Source: CAD feature listing. Evaluate the final solid. Frame: model axes, mm. A direction names the side the tool comes from. Give positions to 0.01 mm unless a question says otherwise; leave off trailing zeros. Loops run counter-clockwise (first coordinate to the right, second up) from the corner with the lowest first, then second, coordinate; pieces in that order, holes last. Notation, with made-up numbers: M 82.25,65.5 L 94.25,65.5 A25 ccw 94.25,98.5 Z; hole C -2,63 d1. An arc over 180 degrees is marked long. Put each result on its own line as item: value.
from build123d import *

# Parameters (mm, degrees)
BOSS_EXTRUDE1_DEPTH = 5
SKETCH5_R           = 2
CUT_EXTRUDE1_DEPTH  = 1.5
SKETCH2_W           = 3
SKETCH2_H           = 3
CUT_EXTRUDE2_DEPTH  = 10


with BuildPart() as part:
    # Sketch1 → Boss-Extrude1 (new body)
    with BuildSketch(Plane.XY):
        with BuildLine():
            ThreePointArc((-10.997222353, 0.247207602), (-0.699194891, -10.977755935), (10.939721705, -1.149999502))
            ThreePointArc((10.939721705, -1.149999502), (10.984920466, -0.575788859), (11.000000502, 4.98e-07))
            ThreePointArc((11.000000502, 4.98e-07), (10.991774906, 0.425318543), (10.967110422, 0.850000498))
            ThreePointArc((10.967110422, 0.850000498), (-0.301772264, 10.995860878), (-10.997222353, 0.247207602))
        make_face()
        with BuildLine():
            ThreePointArc((4.98e-07, -9.049999502), (1.050000497, -7.999999502), (4.96e-07, -6.949999502))
            ThreePointArc((4.96e-07, -6.949999502), (-1.049999502, -7.999999503), (4.98e-07, -9.049999502))
        make_face(mode=Mode.SUBTRACT)
        with BuildLine():
            ThreePointArc((8.000000496, 1.050000498), (6.950000497, 4.97e-07), (8.000000498, -1.049999502))
            ThreePointArc((8.000000498, -1.049999502), (9.050000498, 4.98e-07), (8.000000496, 1.050000498))
        make_face(mode=Mode.SUBTRACT)
        with BuildLine():
            ThreePointArc((4.96e-07, 9.050000498), (-1.049999503, 8.000000497), (4.98e-07, 6.950000498))
            ThreePointArc((4.98e-07, 6.950000498), (1.050000498, 8.000000498), (4.96e-07, 9.050000498))
        make_face(mode=Mode.SUBTRACT)
        with BuildLine():
            ThreePointArc((-9.049999498, -9.4808e-05), (-8.742427926, -0.742495317), (-7.999999502, -1.049999502))
            ThreePointArc((-7.999999502, -1.049999502), (-6.949999502, 4.95e-07), (-7.999999497, 1.050000498))
            ThreePointArc((-7.999999497, 1.050000498), (-8.742495315, 0.742428924), (-9.049999498, -9.4808e-05))
        make_face(mode=Mode.SUBTRACT)
    extrude(amount=BOSS_EXTRUDE1_DEPTH)

    # Sketch5 → Cut-Extrude1 (cut)
    with BuildSketch(Plane.XY.offset(5)):
        with Locations((8.000000497, 4.98e-07)):
            Circle(SKETCH5_R)
        with Locations((4.97e-07, -7.999999502)):
            Circle(SKETCH5_R)
        with Locations((-7.999999502, 4.98e-07)):
            Circle(SKETCH5_R)
        with Locations((4.97e-07, 8.000000498)):
            Circle(SKETCH5_R)
    extrude(amount=-CUT_EXTRUDE1_DEPTH, mode=Mode.SUBTRACT)

    # Sketch2 → Cut-Extrude2 (cut)
    with BuildSketch(Plane.XY.offset(5)):
        Rectangle(SKETCH2_W, SKETCH2_H)
    extrude(amount=-CUT_EXTRUDE2_DEPTH, mode=Mode.SUBTRACT)


solid = part.part
1. Section query A-A (z = 4.45). Output: boundary loops of the cut face in (x, y), plus the area to 3 significant figures.
Found:
outline: C 0,0 d22; hole C -8,0 d4; hole C 0,-8 d4; hole C 0,8 d4; hole M -1.5,-1.5 L 1.5,-1.5 L 1.5,1.5 L -1.5,1.5 Z; hole C 8,0 d4
area: 321 mm^2
2. Material intervals for line 1 (Y direction, x = 0, z = 4.15); line 2 (X direction, y = -0.5, z = 4.35); line 3 (Y direction, x = 8, z = 4.3), sorted ascending. Write a range as from..to.
Found:
line 1: -11..-10, -6..-1.5, 1.5..6, 10..11
line 2: -10.99..-9.94, -6.06..-1.5, 1.5..6.06, 9.94..10.99
line 3: -7.55..-2, 2..7.55
3. Section query B-B (y = 8.5). Output: boundary loops of the cut face in (x, z), plus the area to 3 significant figures.
Found:
outline: M -6.98,0 L -0.92,0 L -0.92,3.5 L -1.94,3.5 L -1.94,5 L -6.98,5 Z; M 0.92,0 L 6.98,0 L 6.98,5 L 1.94,5 L 1.94,3.5 L 0.92,3.5 Z
area: 57.5 mm^2
4. Section query D-D (y = 0.5). Output: boundary loops of the cut face in (x, z), plus the area to 3 significant figures.
Found:
outline: M -10.99,0 L -8.92,0 L -8.92,3.5 L -9.94,3.5 L -9.94,5 L -10.99,5 Z; M -7.08,0 L -1.5,0 L -1.5,5 L -6.06,5 L -6.06,3.5 L -7.08,3.5 Z; M 1.5,0 L 7.08,0 L 7.08,3.5 L 6.06,3.5 L 6.06,5 L 1.5,5 Z; M 8.92,0 L 10.99,0 L 10.99,5 L 9.94,5 L 9.94,3.5 L 8.92,3.5 Z
area: 70.3 mm^2
5. Draft query along X for faces 1 (the flat face through (0, -2, 5)), 2 (the cylindrical face through (-6.153, -0.766, 4.26)). Return one class per face: pulls with the +X half, pulls with the -X half, needs draft (parallel to the pull), parting line crosses it, or undercut.
Found:
face 1: needs draft
face 2: undercut
6. Contact query for flat-ended pins moving along their axis: P1, Ø2, axis at x = 1, z = 0.5, coming from the -Y side; P2, Ø3, axis at y = -3.5, z = 3.5, coming from the -X side; P3, Ø2.5, axis at x = 0, y = 8, coming from the +Z side. Output: stop coordinate, or through.
Found:
P1: y = -11
P2: x = -10.82
P3: z = 3.5
7. Access query for faces 3 (the flat face through (0, -2, 0)), 4 (the flat face through (1, 7, 3.5)), 5 (the flat face through (0, 1.5, 3)). Directions: +Z, -Z, +X, -X, +Y, -Y. A direction counts if a zero-diameter tool reaches every point of the face in a straight line with its end or side. Return the directions, or none.
Found:
face 3: -Z, +X, -X, +Y, -Y
face 4: +Z
face 5: +Z, -Z
